Work out the finished part from the listing and answer in its coordinate system (mm). A direction names the side the tool comes from. Give positions to 0.01 mm unless a question says otherwise; leave off trailing zeros. Loops run counter-clockwise (first coordinate to the right, second up) from the corner with the lowest first, then second, coordinate; pieces in that order, holes last. Notation, with made-up numbers: M -10.75,-6.75 L 22.25,-6.75 A24 cw 22.25,11.25 Z; hole C 70,18 d9. An arc over 180 degrees is marked long. Answer as a JSON object with one key per item and string values. Group by question number.
```python
from build123d import *


with BuildPart() as f1:
    # F0 (on Top) → F1 (revolve)
    with BuildSketch(Plane.XY):
        with BuildLine():
            ThreePointArc((0, 22.7203), (-0.818344, 24.695956), (-2.794, 25.5143))
            Line((-2.794, 25.5143), (-19.05, 25.5143))
            Line((-19.05, 25.5143), (-16.271875, 22.736175))
            Line((-16.271875, 22.736175), (-3.921125, 22.736175))
            ThreePointArc((-3.921125, 22.736175), (-3.112902, 22.401398), (-2.778125, 21.593175))
            Line((-2.778125, 21.593175), (-2.778125, 17.4625))
            Line((-2.778125, 17.4625), (0, 17.4625))
            Line((0, 17.4625), (0, 22.7203))
        make_face()
    revolve(axis=Axis((-9.525, 0, 0), (-1, 0, 0)))


solid = f1.part
```
Item 1: A cutting plane is placed at A-A (y = 0). Determine the outline of the cut face in (x, z), and give its area (3 significant figures).
Item 2: Given pin 1 Ø3 at (x, y) = (-9.5, -11) entering from -Z; pin 2 Ø4 at (x, y) = (-9.5, -14.5) entering from -Z; pin 3 Ø13 at (y, z) = (6, -5.5) entering from -X; pin 4 Ø6 at (x, y) = (-11, 2.5) entering from +Z, each flat-ended and moving along its own axis, determine where each tip first touches the part or whether it passes through.
Item 3: A cutting plane is placed at D-D (x = -2). Determine the outline of the cut face in (y, z) (1 decimal).
Item 4: Find the intervals of material crossed by probe 1 along Y at (x, z) = (-9, 0); probe 2 along Z at (x, y) = (-14.5, 0.5); probe 3 along Z at (x, y) = (-8.25, -17), in increasing order. Write a range as [from, to].
Item 5: A cutting plane is placed at C-C (x = -8). Determine the outline of the cut face in (y, z), and give its area (3 significant figures).
Item 6: A tool of negligible diameter and unlimited length cuts with its end or side. For faces 1 (the cylindrical face through (-10.01, -18.043, 13.835)), 2 (the cylindrical face through (-1.37, -13.858, 10.626)), from which of +Z, -Z, +X, -X, +Y, -Y can it reach the whole face along a straight path? Write none if from no direction.
The answers:
{
 "1": {"outline": "M -19.05,-25.51 L -2.79,-25.51 A2.79 ccw 0,-22.72 L 0,-17.46 L -2.78,-17.46 L -2.78,-21.59 A1.14 cw -3.92,-22.74 L -16.27,-22.74 Z; M -19.05,25.51 L -16.27,22.74 L -3.92,22.74 A1.14 cw -2.78,21.59 L -2.78,17.46 L 0,17.46 L 0,22.72 A2.79 ccw -2.79,25.51 Z", "area": "125 mm^2"},
 "2": {"pin 1": "stops at z = -23.68", "pin 2": "stops at z = -22.24", "pin 3": "passes through", "pin 4": "stops at z = 25.51"},
 "3": {"outline": "C 0,0 d50.8; hole C 0,0 d34.9"},
 "4": {"probe 1": "y = [-25.51, -22.74], [22.74, 25.51]", "probe 2": "z = [-25.51, -22.73], [22.73, 25.51]", "probe 3": "z = [-19.03, -15.1], [15.1, 19.03]"},
 "5": {"outline": "C 0,0 d51.03; hole C 0,0 d45.47", "area": "421 mm^2"},
 "6": {"face 1": "-X", "face 2": "+X, -X"}
}
